Source: CAD feature listing. Evaluate the final solid. Frame: model axes, mm. Round coordinates to 2 decimals unless told otherwise and drop trailing zeros.
Item 1: First-contact query: P1, Ø5, axis at x = -2.5, z = -134, coming from the +Y side; P2, Ø0.8, axis at y = 14.5, z = -99, coming from the +X side; P3, Ø3, axis at y = 2, z = 61.5, coming from the +X side; P4, Ø12, axis at x = -6.5, y = 3, coming from the -Z side. Flat tips, straight axial feed; report the tip coordinate or a pass-through.
Item 2: Section query A-A on z = 97. Give the number of separate pieces and of enclosed holes in the cut face, then the cut area to 3 significant figures.
Item 3: Ray query, L1, parallel to X at y = 12, z = -92; L2, parallel to X at y = 10.5, z = -32. Return the intervals inside material, ascending.
```python
from build123d import *

# Parameters (mm, degrees)
F1_DEPTH = 261.5


with BuildPart() as f1:
    # F0 (on Top) → F1 (new body, symmetric)
    with BuildSketch(Plane.XY):
        with BuildLine():
            Line((-5.1, 14), (-5.1, 15))
            Line((-5.1, 15), (-12.5, 15))
            ThreePointArc((-12.5, 15), (-14.267767, 14.267767), (-15, 12.5))
            Line((-15, 12.5), (-15, 5.1))
            Line((-15, 5.1), (-14, 5.1))
            Line((-14, 5.1), (-14, 4.1))
            Line((-14, 4.1), (-13, 4.1))
            Line((-13, 4.1), (-13, 8.25))
            Line((-13, 8.25), (-9.7, 8.25))
            Line((-9.7, 8.25), (-5.8, 4.35))
            Line((-5.8, 4.35), (-5.8, 0.5))
            Line((-5.8, 0.5), (-5.5, 0))
            Line((-5.5, 0), (-3.4, 0))
            ThreePointArc((-3.4, 0), (-2.404163, 2.404163), (0, 3.4))
            Line((0, 3.4), (0, 5.5))
            Line((0, 5.5), (-0.5, 5.8))
            Line((-0.5, 5.8), (-4.35, 5.8))
            Line((-4.35, 5.8), (-8.25, 9.7))
            Line((-8.25, 9.7), (-8.25, 13))
            Line((-8.25, 13), (-4.1, 13))
            Line((-4.1, 13), (-4.1, 14))
            Line((-4.1, 14), (-5.1, 14))
        make_face()
        with BuildLine():
            ThreePointArc((-13, 12.5), (-12.853553, 12.853553), (-12.5, 13))
            Line((-12.5, 13), (-10.75, 13))
            ThreePointArc((-10.75, 13), (-10.396447, 12.853553), (-10.25, 12.5))
            Line((-10.25, 12.5), (-10.25, 10.75))
            ThreePointArc((-10.25, 10.75), (-10.396447, 10.396447), (-10.75, 10.25))
            Line((-10.75, 10.25), (-12.5, 10.25))
            ThreePointArc((-12.5, 10.25), (-12.853553, 10.396447), (-13, 10.75))
            Line((-13, 10.75), (-13, 12.5))
        make_face(mode=Mode.SUBTRACT)
    extrude(amount=F1_DEPTH, both=True)

    # F2: F1 across face


with BuildPart() as f1_1:
    add(f1.part)
    add(f1.part.mirror(Plane(origin=(0, 4.45, 0), x_dir=(0, 1, 0), z_dir=(1, 0, 0))))

    # F3: F1 across face


with BuildPart() as f1_2:
    add(f1_1.part)
    add(f1_1.part.mirror(Plane(origin=(-4.45, 0, 0), x_dir=(1, 0, 0), z_dir=(0, -1, 0))))


solid = f1_2.part
```
Data:
1. P1: stops at y = 14
1. P2: stops at x = 14.42
1. P3: stops at x = 5.8
1. P4: stops at z = -261.5
2. separate pieces: 1
2. enclosed holes: 5
2. area: 340 mm2
3. L1: x = -15 to -13, -10.25 to -8.25, 8.25 to 10.25, 13 to 15
3. L2: x = -15 to -12.93, -10.32 to -8.25, 8.25 to 10.32, 12.93 to 15
